```python
from build123d import *

# Parameters (mm, degrees)
F1_DEPTH    = 2.54
F3_DEPTH    = 86.106
F5_DEPTH    = 95.25
F7_DEPTH    = 55.626
F8_R        = 63.189953
F9_DEPTH    = 2.54
F10_R       = 4.593675
F11_DEPTH   = 25.4
F9_FACE_R   = 63.189953
F9_FACE_R_2 = 4.593675
F12_DEPTH   = 7.62


with BuildPart() as f1:
    # F0 (on Top) → F1 (new body)
    with BuildSketch(Plane.XY):
        Polygon((9.110871, 18.553045), (0, 18.553045), (-9.110871, 18.553045), (-28.326523, 54.002609), (-34.952607, 57.315651), (-47.210872, 12.92087), (-42.903915, -10.933043), (-7.785654, -47.707826), (0, -50.358262), (7.785654, -47.707826), (42.903915, -10.933043), (47.210872, 12.92087), (34.952607, 57.315651), (28.326523, 54.002609), align=None)
    extrude(amount=F1_DEPTH)

    # F2 (on Top) → F3 (cut)
    with BuildSketch(Plane.XY):
        Polygon((-5.466522, -9.93913), (-8.779565, -3.644348), (-16.399564, 0), (-30.645652, 4.638261), (-22.363044, -3.975652), align=None)
        Polygon((8.779565, -3.644348), (5.466522, -9.93913), (22.363044, -3.975652), (30.645652, 4.638261), (16.399564, 0), align=None)
    extrude(amount=F3_DEPTH, mode=Mode.SUBTRACT)

    # F4 (on Top) → F5 (cut)
    with BuildSketch(Plane.XY):
        Polygon((-36.940437, -13.583479), (-33.296086, -6.294783), (-36.940437, 0), (-36.940437, -5.632174), align=None)
        Polygon((-29.651739, -22.197392), (-26.670001, -11.926956), (-29.651739, -7.288696), (-32.633476, -12.589565), align=None)
        Polygon((-23.827148, -27.621334), (-21.700436, -14.577392), (-25.51044, -22.197392), align=None)
        Polygon((-14.765322, -21.278939), (-17.724782, -22.197392), (-17.730825, -31.802197), (-12.928419, -22.197392), align=None)
        Polygon((-7.785654, -27.166957), (-12.423914, -30.148696), (-4.803916, -45.388699), align=None)
        Polygon((12.423914, -30.148696), (7.785654, -27.166957), (4.803916, -45.388699), align=None)
        Polygon((17.724782, -19.799208), (12.928419, -22.197392), (17.730825, -31.802197), (17.724782, -22.197392), align=None)
        Polygon((21.700436, -14.577392), (23.827148, -27.621334), (25.51044, -22.197392), align=None)
        Polygon((26.670001, -11.926956), (29.651739, -22.197392), (32.633476, -12.589565), (29.651739, -7.288696), align=None)
        Polygon((33.296086, -6.294783), (36.940437, -13.583479), (36.940437, -5.632174), (36.940437, 0), align=None)
        Polygon((-5.071647, -26.487922), (-4.472611, -30.148696), (-1.531945, -40.594514), (-3.24126, -30.148696), align=None)
        Polygon((3.24126, -30.148696), (1.531945, -40.594514), (4.472611, -30.148696), (5.071647, -26.487922), align=None)
    extrude(amount=F5_DEPTH, mode=Mode.SUBTRACT)

    # F6 (on Top) → F7 (cut)
    with BuildSketch(Plane.XY):
        Polygon((-2.816088, -21.203479), (-2.816088, -10.601739), (-5.797826, -16.896522), align=None)
        Polygon((2.816088, -10.601739), (2.816088, -21.203479), (5.797826, -16.896522), align=None)
    extrude(amount=F7_DEPTH, mode=Mode.SUBTRACT)

    # F8 (on face) → F9 (join)
    with BuildSketch(Plane(origin=(0, 0, 0), x_dir=(1, 0, 0), z_dir=(0, 0, -1))):
        Circle(F8_R)
    extrude(amount=F9_DEPTH)

    # F10 (on face) → F11 (cut)
    with BuildSketch(Plane.XY):
        with Locations((0, 54.996524)):
            Circle(F10_R)
    extrude(amount=-F11_DEPTH, mode=Mode.SUBTRACT)

    # F9_face (on face) → F12 (join)
    with BuildSketch(Plane(origin=(0, -0.292187, -2.54), x_dir=(1, 0, 0), z_dir=(0, 0, -1))):
        with Locations((0, -0.292187)):
            Circle(F9_FACE_R)
        with Locations((0, -55.288711)):
            Circle(F9_FACE_R_2, mode=Mode.SUBTRACT)
    extrude(amount=F12_DEPTH)


solid = f1.part
```
Verification items for the finished model (mm, model axes). A direction names the side the tool comes from. Round coordinates to 2 decimals unless told otherwise and drop trailing zeros. Write each loop counter-clockwise with the first axis right and the second up, starting at its lowest first coordinate (ties: lowest second). Pieces come first, ordered by that corner, then holes. Notation, with made-up numbers: (17.25, -39) - (23.25, -39) arc R20 cw to (23.25, -35) - close; hole circle Ø3 at (9.5, 10.5). An arc over 180 degrees is marked (long way). Answer as a JSON object with one key per item and string values. Group by question number.
Q1. Section check A-A, the plane z = -2.5. Enter the section's corners in (x, y), plus the area to 3 significant figures.
Q2. Mould release check, pull along X, two halves, no side actions. Record for faces 1 (the flat face through (45.027, 0.827, 1.252)), 2 (the flat face through (-36, -7, 0)), 3 (the flat face through (-30, -15, 0)): released by +X, released by -X, zero draft, split by the parting line, or undercut.
Q3. Section check B-B, the plane x = -52.5. Enter the section's corners in (y, z), plus the area to 3 significant figures.
Q4. Thickness scan on line 1 (Y direction, x = 0, z = -4.5); line 2 (Y direction, x = 34, z = 1); line 3 (Z direction, x = -37, y = -18). Record the ranges inside material, lowest first.
Q5. Section check C-C, the plane x = 51.5. Enter the section's corners in (y, z).
Q6. Go/stop test with flat-tipped pins: pin 1 Ø6.5 at (x, y) = (-33, 55) entering from -Z; pin 2 Ø0.8 at (y, z) = (-7, 1.5) entering from +X; pin 3 Ø10.5 at (x, y) = (0, 55) entering from +Z; pin 4 Ø2 at (y, z) = (-22.5, -8) entering from -X. Record where each tip stops, or that it passes through.
Q7. Tool access check on faces 4 (the flat face through (4, -16, 0)), 5 (the flat face through (0, 46, 0)), 6 (the cylindrical face through (2.12, 59.07, -5.01)). Record the directions out of +Z, -Z, +X, -X, +Y, -Y that give a thin tool (end or side, any length) a straight path to the whole face; none if there is none.
Found:
{
 "1": {"outline": "circle Ø126.38 at (0, 0); hole circle Ø9.19 at (0, 55)", "area": "12,500 mm^2"},
 "2": {"face 1": "released by +X", "face 2": "undercut", "face 3": "undercut"},
 "3": {"outline": "(-35.17, -10.16) - (35.17, -10.16) - (35.17, 0) - (-35.17, 0) - close", "area": "715 mm^2"},
 "4": {"line 1": "y = -63.19 to 50.4, 59.59 to 63.19", "line 2": "y = -20.26 to -7.7, -5.08 to 56.84", "line 3": "z = -10.16 to 0"},
 "5": {"outline": "(-36.62, -10.16) - (36.62, -10.16) - (36.62, 0) - (-36.62, 0) - close"},
 "6": {"pin 1": "stops at z = -10.16", "pin 2": "stops at x = 43.69", "pin 3": "stops at z = 0", "pin 4": "stops at x = -59.42"},
 "7": {"face 4": "+Z", "face 5": "+Z, +Y", "face 6": "+Z, -Z"}
}
